The listing builds one solid part. Answer for the finished solid, in the listing's coordinates (mm). Face numbers are marked on the shaded views. A direction names the side the tool comes from. Coordinates: 2 decimals unless noted, no trailing zeros. Loops run counter-clockwise (first coordinate to the right, second up) from the corner with the lowest first, then second, coordinate; pieces in that order, holes last. Notation, with made-up numbers: (14, -27.5) - (58, -27.5) arc R24 ccw to (58, -14.5) - close; hole circle Ø5 at (49, 42). An arc over 180 degrees is marked (long way). Put each result on its own line as item: value.
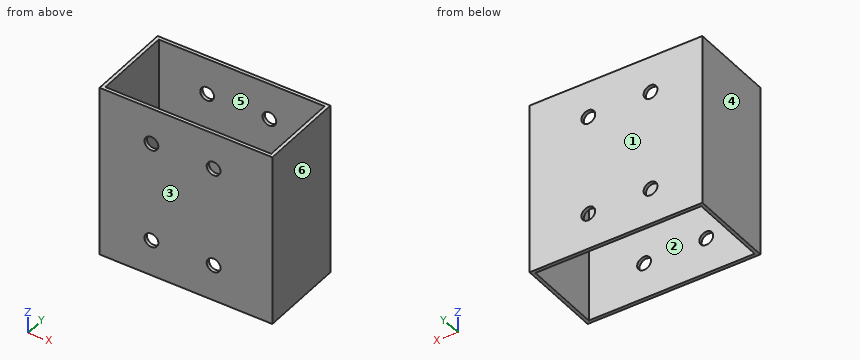
```python
from build123d import *

# Parameters (mm, degrees)
SKETCH_1_W          = 50
SKETCH_1_H          = 25
SKETCH_1_W_2        = 48
SKETCH_1_H_2        = 23
EXTRUDE_1_DEPTH     = 50
SKETCH_2_R          = 2
CUT_EXTRUDE_1_DEPTH = 50


with BuildPart() as part:
    # 草图1 → 凸台-拉伸1 (new body)
    with BuildSketch(Plane.XY):
        with Locations((25, 12.5)):
            Rectangle(SKETCH_1_W, SKETCH_1_H)
        with Locations((25, 12.5)):
            Rectangle(SKETCH_1_W_2, SKETCH_1_H_2, mode=Mode.SUBTRACT)
    extrude(amount=EXTRUDE_1_DEPTH)

    # 草图2 → 切除-拉伸1 (cut)
    with BuildSketch(Plane(origin=(0, 25, 0), x_dir=(1, 0, 0), z_dir=(0, 1, 0))):
        with Locations(Location((15, -10.5, 0), (0, 0, 270))):
            Circle(SKETCH_2_R)
        with Locations(Location((33, -10.5, 0), (0, 0, 270))):
            Circle(SKETCH_2_R)
        with Locations(Location((33, -39.5, 0), (0, 0, 270))):
            Circle(SKETCH_2_R)
        with Locations(Location((15, -39.5, 0), (0, 0, 270))):
            Circle(SKETCH_2_R)
    extrude(amount=-CUT_EXTRUDE_1_DEPTH, mode=Mode.SUBTRACT)


solid = part.part
```
1) For the marked faces 1 and 2, determine the directions among +Z, -Z, +X, -X, +Y, -Y from which every point of the face is accessible in a straight line to the end or side of a thin tool.
Found:
face 1: +Z, -Z, +X, -X, +Y
face 2: +Z, -Z
2) For a pull along X with two mould halves and no side action, classify the marked faces 3, 4, 5 and 6 as pulls with the +X half, pulls with the -X half, needs draft (parallel to the pull), parting line crosses it, or undercut.
Found:
face 3: needs draft
face 4: pulls with the -X half
face 5: undercut
face 6: pulls with the +X half
3) Each of these flat-tipped pins is pushed along its axis until it touches: pin 1 (2.5 mm diameter, centred on x = 15, z = 39.5, fed in from -Y); pin 2 (6.5 mm diameter, centred on x = 15, z = 10.5, fed in from +Y). Where does it stop, or does it pass through?
Found:
pin 1: passes through
pin 2: stops at y = 25
4) The part is cut by section D-D (z = 17). Give the vertices of the cut face in (x, y), and give its area (3 significant figures).
Found:
outline: (0, 0) - (50, 0) - (50, 25) - (0, 25) - close; hole (1, 1) - (49, 1) - (49, 24) - (1, 24) - close
area: 146 mm^2
5) The part is cut by section C-C (y = 22). Give the vertices of the cut face in (x, z), and give its area (3 significant figures).
Found:
outline: (0, 0) - (1, 0) - (1, 50) - (0, 50) - close; (49, 0) - (50, 0) - (50, 50) - (49, 50) - close
area: 100 mm^2
6) The part is cut by section A-A (x = 15). Give the vertices of the cut face in (y, z), and give its area (3 significant figures).
Found:
outline: (0, 0) - (1, 0) - (1, 8.5) - (0, 8.5) - close; (0, 12.5) - (1, 12.5) - (1, 37.5) - (0, 37.5) - close; (0, 41.5) - (1, 41.5) - (1, 50) - (0, 50) - close; (24, 0) - (25, 0) - (25, 8.5) - (24, 8.5) - close; (24, 12.5) - (25, 12.5) - (25, 37.5) - (24, 37.5) - close; (24, 41.5) - (25, 41.5) - (25, 50) - (24, 50) - close
area: 84.0 mm^2
7) Straight lines are drawn through the part: L1, parallel to X at y = 0.2, z = 10.5; L2, parallel to Y at x = 28, z = 10.5; L3, parallel to X at y = 22.5, z = 6.5. For each, find the intervals that lie inside material, in ascending order. Write a range as [from, to].
Found:
L1: x = [0, 13], [17, 31], [35, 50]
L2: y = [0, 1], [24, 25]
L3: x = [0, 1], [49, 50]
8) The part is cut by section B-B (z = 10.5). Give the vertices of the cut face in (x, y).
Found:
outline: (0, 0) - (13, 0) - (13, 1) - (1, 1) - (1, 24) - (13, 24) - (13, 25) - (0, 25) - close; (17, 0) - (31, 0) - (31, 1) - (17, 1) - close; (17, 24) - (31, 24) - (31, 25) - (17, 25) - close; (35, 0) - (50, 0) - (50, 25) - (35, 25) - (35, 24) - (49, 24) - (49, 1) - (35, 1) - close
